from build123d import *

# Parameters (mm, degrees)
F0_R     = 20
F1_DEPTH = 15
F2_W     = 40
F2_H     = 2.5
F3_DEPTH = 15
F4_R     = 10
F5_DEPTH = 25


with BuildPart() as f1:
    # F0 (on Top) → F1 (new body)
    with BuildSketch(Plane.XY):
        Circle(F0_R)
    extrude(amount=F1_DEPTH)

    # F2 (on Top) → F3 (join)
    with BuildSketch(Plane.XY):
        with Locations((20, 1.25)):
            Rectangle(F2_W, F2_H)
        with Locations((20, -1.25)):
            Rectangle(F2_W, F2_H)
    extrude(amount=F3_DEPTH)

    # F4 (on Top) → F5 (join)
    with BuildSketch(Plane.XY):
        Circle(F4_R)
    extrude(amount=F5_DEPTH)


solid = f1.part
Geometry check sheet. Reference: the model listing, model coordinates, mm. A direction names the side the tool comes from. Round coordinates to 2 decimals unless told otherwise and drop trailing zeros. Write each loop counter-clockwise with the first axis right and the second up, starting at its lowest first coordinate (ties: lowest second). Pieces come first, ordered by that corner, then holes.
Item 1: Section check A-A (x = 0). Record the boundary of the cut face in (y, z), plus the area to 3 significant figures.
Determined:
outline: (-20, 0) - (20, 0) - (20, 15) - (10, 15) - (10, 25) - (-10, 25) - (-10, 15) - (-20, 15) - close
area: 800 mm2
Item 2: Section check C-C (z = 4.5). Record the boundary of the cut face in (x, y), plus the area to 3 significant figures.
Determined:
outline: (19.84, -2.5) - (40, -2.5) - (40, 2.5) - (19.84, 2.5) arc R20 ccw (long way) to start
area: 1,360 mm2
Item 3: Access from +Z, -Z, +X, -X, +Y, -Y to the whole of each face (thin tool, end or side, straight path). Record for faces 1 (the face through (30, 2.5, 7)), 2 (the face through (30, -2.5, 7)), 3 (the face through (-19.982, 0.844, 7.395)), 4 (the face through (3, 0, 0)), 5 (the face through (10, -4, 15)).
Determined:
face 1: +Z, -Z, +X, +Y
face 2: +Z, -Z, +X, -Y
face 3: +Z, -Z
face 4: -Z, +X, -X, +Y, -Y
face 5: +Z
Item 4: Section check D-D (x = 23.5). Record the boundary of the cut face in (y, z), plus the area to 3 significant figures.
Determined:
outline: (-2.5, 0) - (2.5, 0) - (2.5, 15) - (-2.5, 15) - close
area: 75.0 mm2
Item 5: Material ranges on line 1 along Z through (x, y) = (-8.5, 13.5); line 2 along Y through (x, z) = (28.5, 3.75); line 3 along X through (y, z) = (-0.5, 9), recorded low to high.
Determined:
line 1: z = 0 to 15
line 2: y = -2.5 to 2.5
line 3: x = -19.99 to 40
Item 6: Section check B-B (y = 0). Record the boundary of the cut face in (x, z), plus the area to 3 significant figures.
Determined:
outline: (-20, 0) - (40, 0) - (40, 15) - (10, 15) - (10, 25) - (-10, 25) - (-10, 15) - (-20, 15) - close
area: 1,100 mm2
Item 7: Go/stop test with flat-tipped pins: pin 1 Ø3 at (y, z) = (-13, 10.5) entering from -X; pin 2 Ø5 at (y, z) = (8, 10.5) entering from -X; pin 3 Ø7.5 at (x, z) = (30.5, 6) entering from -Y. Record where each tip stops, or that it passes through.
Determined:
pin 1: stops at x = -16.36
pin 2: stops at x = -19.23
pin 3: stops at y = -2.5
